from build123d import *

# Parameters (mm, degrees)
SKETCH1_R               = 22.5
BOSS_EXTRUDE1_DEPTH     = 30
SKETCH2_R               = 7.5
SKETCH2_W               = 3
SKETCH2_H               = 30
SKETCH2_W_2             = 30
SKETCH2_H_2             = 3
CUT_EXTRUDE1_DEPTH      = 10
SKETCH3_W               = 15.299534312
SKETCH3_H               = 14.93812799
BOSS_EXTRUDE2_DEPTH     = 20
CUT_EXTRUDE2_DEPTH      = 20
SKETCH5_R               = 2.5
CUT_EXTRUDE4_DEPTH      = 20
SKETCH10_W              = 15.299534312
SKETCH10_H              = 5
CUT_EXTRUDE5_DEPTH      = 23
CUT_EXTRUDE5_DEPTH_BACK = 11.4
SKETCH11_W              = 15.299534312
SKETCH11_H              = 5
SKETCH11_R              = 2.5
BOSS_EXTRUDE3_DEPTH     = 8
SKETCH13_W              = 10
SKETCH13_H              = 3.47
SKETCH13_W_2            = 5
CUT_EXTRUDE6_DEPTH      = 21


with BuildPart() as part:
    # Sketch1 → Boss-Extrude1 (new body)
    with BuildSketch(Plane.XY):
        Circle(SKETCH1_R)
    extrude(amount=BOSS_EXTRUDE1_DEPTH)

    # Sketch2 → Cut-Extrude1 (cut)
    with BuildSketch(Plane(origin=(0, 0, 0), x_dir=(-1, 0, 0), z_dir=(0, 0, -1))):
        Circle(SKETCH2_R)
        Rectangle(SKETCH2_W, SKETCH2_H)
        Rectangle(SKETCH2_W_2, SKETCH2_H_2)
    extrude(amount=-CUT_EXTRUDE1_DEPTH, mode=Mode.SUBTRACT)

    # Sketch3 → Boss-Extrude2 (add)
    with BuildSketch(Plane.XY.offset(30)):
        Rectangle(SKETCH3_W, SKETCH3_H)
    extrude(amount=BOSS_EXTRUDE2_DEPTH)

    # Sketch4 → Cut-Extrude2 (cut)
    with BuildSketch(Plane.ZY.offset(7.649767156)):
        Polygon((40, 4), (50, 4), (50, 0), (50, -4), (40, -4), (35, -4), (35, 4), align=None)
    extrude(amount=-CUT_EXTRUDE2_DEPTH, mode=Mode.SUBTRACT)

    # Sketch5 → Cut-Extrude4 (cut)
    with BuildSketch(Plane(origin=(0, 7.469063995, 0), x_dir=(1, 0, 0), z_dir=(0, 1, 0))):
        with Locations((0, -45)):
            Circle(SKETCH5_R)
        with BuildLine():
            Line((7.649767156, -50), (7.649767156, -40))
            add(Edge.make_bspline(
                [(0, -50), (7.649767156, -50), (7.649767156, -40)],
                knots=[3.141592654, 3.141592654, 3.141592654, 4.71238898, 4.71238898, 4.71238898], degree=2, weights=[1, 0.707106781, 1]))
            Line((0, -50), (7.649767156, -50))
        make_face()
        with BuildLine():
            Line((-7.649767156, -50), (0, -50))
            add(Edge.make_bspline(
                [(-7.649767156, -40), (-7.649767156, -50), (0, -50)],
                knots=[1.570796327, 1.570796327, 1.570796327, 3.141592654, 3.141592654, 3.141592654], degree=2, weights=[1, 0.707106781, 1]))
            Line((-7.649767156, -40), (-7.649767156, -50))
        make_face()
    extrude(amount=-CUT_EXTRUDE4_DEPTH, mode=Mode.SUBTRACT)

    # Sketch10 → Cut-Extrude5 (cut, two sides)
    with BuildSketch(Plane(origin=(0, 7.469063995, 0), x_dir=(1, 0, 0), z_dir=(0, 1, 0))) as cut_extrude5_sk:
        with Locations((0, -37.5)):
            Rectangle(SKETCH10_W, SKETCH10_H)
        with BuildLine():
            Line((7.649767156, -40), (-7.649767156, -40))
            add(Edge.make_bspline(
                [(-7.649767156, -40), (-7.649767156, -50), (0, -50), (7.649767156, -50), (7.649767156, -40)],
                knots=[4.71238898, 4.71238898, 4.71238898, 6.283185307, 6.283185307, 7.853981634, 7.853981634, 7.853981634], degree=2, weights=[1, 0.707106781, 1, 0.707106781, 1]))
        make_face()
    extrude(amount=CUT_EXTRUDE5_DEPTH, mode=Mode.SUBTRACT)
    extrude(cut_extrude5_sk.sketch, amount=-CUT_EXTRUDE5_DEPTH_BACK, mode=Mode.SUBTRACT)

    # Sketch11 → Boss-Extrude3 (add)
    with BuildSketch(Plane(origin=(0, -4, 0), x_dir=(1, 0, 0), z_dir=(0, 1, 0))):
        with Locations((0, -37.5)):
            Rectangle(SKETCH11_W, SKETCH11_H)
        with BuildLine():
            Line((7.649767156, -40), (-7.649767156, -40))
            add(Edge.make_bspline(
                [(-7.649767156, -40), (-7.649767156, -50), (0, -50), (7.649767156, -50), (7.649767156, -40)],
                knots=[4.71238898, 4.71238898, 4.71238898, 6.283185307, 6.283185307, 7.853981634, 7.853981634, 7.853981634], degree=2, weights=[1, 0.707106781, 1, 0.707106781, 1]))
        make_face()
        with Locations((0, -45)):
            Circle(SKETCH11_R, mode=Mode.SUBTRACT)
    extrude(amount=BOSS_EXTRUDE3_DEPTH)

    # Sketch13 → Cut-Extrude6 (cut)
    with BuildSketch(Plane.ZY.offset(7.649767156)):
        with Locations((45, -5.734063995)):
            Rectangle(SKETCH13_W, SKETCH13_H)
        with Locations((37.5, -5.734063995)):
            Rectangle(SKETCH13_W_2, SKETCH13_H)
    extrude(amount=-CUT_EXTRUDE6_DEPTH, mode=Mode.SUBTRACT)


solid = part.part
The model under review builds one solid part; all positions refer to its coordinate system, in mm. A direction names the side the tool comes from. Round coordinates to 2 decimals unless told otherwise and drop trailing zeros. Write each loop counter-clockwise with the first axis right and the second up, starting at its lowest first coordinate (ties: lowest second). Pieces come first, ordered by that corner, then holes. Notation, with made-up numbers: M 31.25,24 L 71.25,24 A21 ccw 71.25,49 Z; hole C 24.25,1 d3. An arc over 180 degrees is marked long. Answer as CSV lines item,"result". Start each with the question number.
Q1. Tool access review of faces 5 (the face through (0, -6, 35)), 6 (the face through (10.382, -19.961, 14.79)), 7 (the face through (-1.5, -11, 5)): name each direction out of +Z, -Z, +X, -X, +Y, -Y from which nothing blocks a thin tool from reaching the whole face with its end or side.
Q2. Consider section B-B, the plane x = 10.5. Give the boundary of the cut face in (y, z), then the cut area to 3 significant figures.
Q3. Clearance check with flat-ended pins moving along their axes: P1, Ø3, axis at y = -17.5, z = 13.5, coming from the -X side; P2, Ø6, axis at x = 6.5, y = -15.5, coming from the +Z side; P3, Ø6, axis at y = 11.5, z = 6, coming from the +X side. State where each tip first meets the part, or that it passes through.
Q4. The part is to be moulded in two halves that separate along Y. For faces 1 (the face through (0, -15, 5)), 2 (the face through (0, 7.469, 32)), 3 (the face through (10, -5, 0)), 4 (the face through (0, -7.469, 32)), say which applies: +Y half, -Y half, draft (parallel to the pull), parting line (faces both ways), or undercut.
Q5. Consider section A-A, the plane z = 7. Give the boundary of the cut face in (x, y), then the cut area to 3 significant figures.
Q6. Consider section D-D, the plane z = 28. Give the boundary of the cut face in (x, y), then the cut area to 3 significant figures.
Q7. Wall thickness on line 1 along Z through (x, y) = (0, -2); line 2 along Y through (x, z) = (5, 43); line 3 along Y through (x, z) = (13, 5): over which ranges is each line inside the solid? List them lowest first.
Q8. Consider section C-C, the plane y = -11. Give the boundary of the cut face in (x, z), then the cut area to 3 significant figures.
Result set:
1,face 5,"+Z, +X, -X, -Y"
1,face 6,"+Z, -Z"
1,face 7,"-Z"
2,outline,"M -19.9,0 L -1.5,0 L -1.5,10 L 1.5,10 L 1.5,0 L 19.9,0 L 19.9,30 L -19.9,30 Z"
2,area,"1,160 mm²"
3,P1,"stops at x = -15.82"
3,P2,"stops at z = 30"
3,P3,"stops at x = 20.83"
4,face 1,"undercut"
4,face 2,"+Y half"
4,face 3,"draft"
4,face 4,"-Y half"
5,outline,"C 0,0 d45; hole M -15,-1.5 L -7.35,-1.5 A7.5 ccw -1.5,-7.35 L -1.5,-15 L 1.5,-15 L 1.5,-7.35 A7.5 ccw 7.35,-1.5 L 15,-1.5 L 15,1.5 L 7.35,1.5 A7.5 ccw 1.5,7.35 L 1.5,15 L -1.5,15 L -1.5,7.35 A7.5 ccw -7.35,1.5 L -15,1.5 Z"
5,area,"1,320 mm²"
6,outline,"C 0,0 d45"
6,area,"1,590 mm²"
7,line 1,"z = 10 to 42.5, 47.5 to 50"
7,line 2,"y = -4 to 4"
7,line 3,"y = -18.36 to -1.5, 1.5 to 18.36"
8,outline,"M -19.63,0 L -1.5,0 L -1.5,10 L 1.5,10 L 1.5,0 L 19.63,0 L 19.63,30 L -19.63,30 Z"
8,area,"1,150 mm²"
